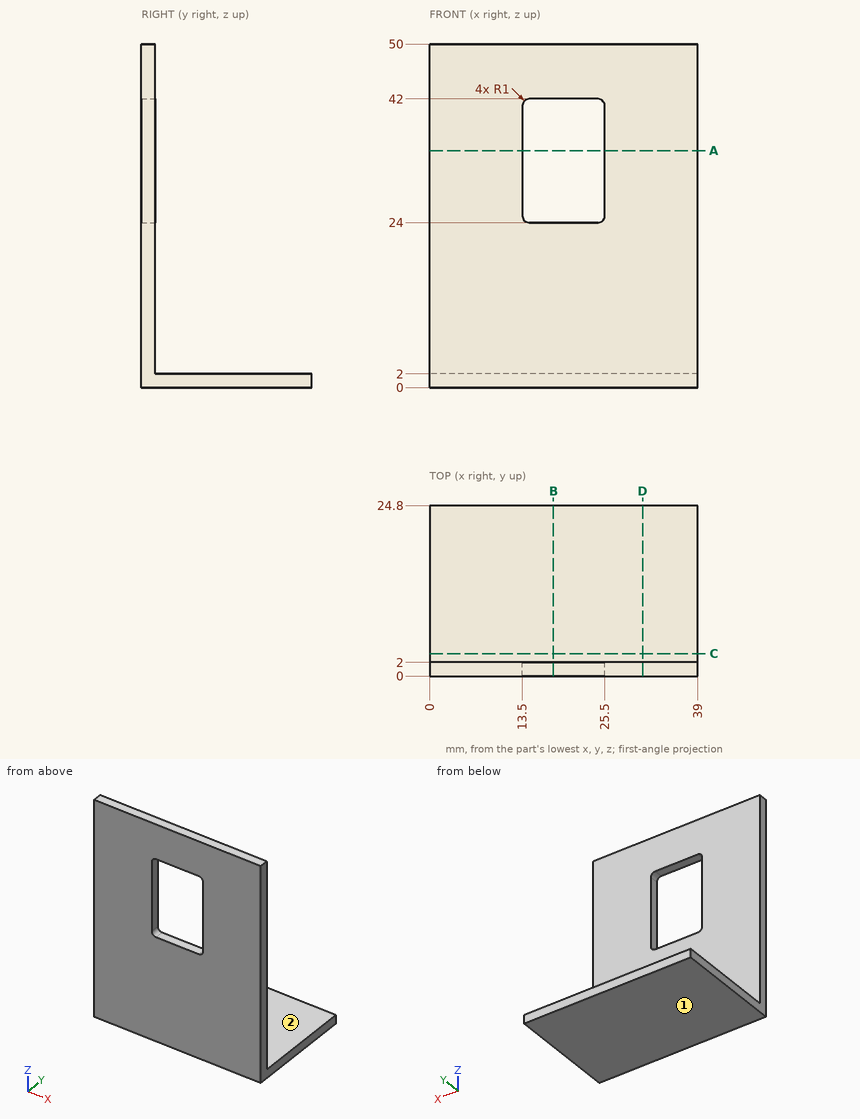
Verification items for this drawing (mm, ordinates from the low corner). A direction names the side the tool comes from. Coordinates: 2 decimals unless noted, no trailing zeros. Order: outer loops, then holes, each group sorted by start corner. A loop starts at its lowest first (then second) coordinate and runs counter-clockwise, first axis right, second up. Notation, with made-up numbers: (85.25, -38) - (133.25, -38) arc R9 ccw to (133.25, -29) - close; hole circle Ø6 at (2, 37). An arc over 180 degrees is marked (long way). Answer as a JSON object with one key per item and string values. Group by question number.
Item 1: Sectioned sample at A-A, the plane z = 34.5. Record the cut outline in (x, y), and give its area (3 significant figures).
Item 2: Scan line: probe 1 along Y at (x, z) = (10.5, 10). Record every from-to range of solid material in increasing order.
Item 3: Sectioned sample at B-B, the plane x = 18. Record the cut outline in (y, z).
Item 4: Sectioned sample at C-C, the plane y = 3.25. Record the cut outline in (x, z), and give its area (3 significant figures).
Item 5: Sectioned sample at D-D, the plane x = 31. Record the cut outline in (y, z), and give its area (3 significant figures).
Item 6: Tool access check on the marked faces 1 and 2. Record the directions out of +Z, -Z, +X, -X, +Y, -Y that give a thin tool (end or side, any length) a straight path to the whole face; none if there is none.
Item 7: Depth check by flat-ended pin: pin 1 Ø12 at (x, y) = (19, 13) entering from +Z; pin 2 Ø10 at (x, z) = (13.5, 16.5) entering from +Y. Enter the tip coordinate at first touch or a pass-through.
Resolved:
{
 "1": {"outline": "(0, 0) - (13.5, 0) - (13.5, 2) - (0, 2) - close; (25.5, 0) - (39, 0) - (39, 2) - (25.5, 2) - close", "area": "54.0 mm^2"},
 "2": {"probe 1": "0 to 2"},
 "3": {"outline": "(0, 0) - (24.8, 0) - (24.8, 2) - (2, 2) - (2, 24) - (0, 24) - close; (0, 42) - (2, 42) - (2, 50) - (0, 50) - close"},
 "4": {"outline": "(0, 0) - (39, 0) - (39, 2) - (0, 2) - close", "area": "78.0 mm^2"},
 "5": {"outline": "(0, 0) - (24.8, 0) - (24.8, 2) - (2, 2) - (2, 50) - (0, 50) - close", "area": "146 mm^2"},
 "6": {"face 1": "-Z, +X, -X, +Y, -Y", "face 2": "+Z, +X, -X, +Y"},
 "7": {"pin 1": "z = 2", "pin 2": "y = 2"}
}
